Verification items for the finished model (mm, model axes). A direction names the side the tool comes from. Give positions to 0.01 mm unless a question says otherwise; leave off trailing zeros. One line per question, with ' | ' between items. Start each with the question number.
Q1. Go/stop test with flat-tipped pins: pin 1 (10 mm diameter, centred on y = 27.5, z = 22, fed in from +X); pin 2 (3 mm diameter, centred on x = -14.14, y = 14.14, fed in from +Z); pin 3 (1 mm diameter, centred on x = -38, z = 39.5, fed in from +Y). Record where each tip stops, or that it passes through.
Q2. Section check A-A on z = 7. Give the number of separate pieces and of enclosed holes in the cut face, plus the area to 3 significant figures.
Q3. Access from +Z, -Z, +X, -X, +Y, -Y to the whole of each face (thin tool, end or side, straight path). Record for faces 1 (the cylindrical face through (-47.44, 0.07, 42.35)), 2 (the cylindrical face through (14.985, 0.66, 12.325)), 3 (the flat face through (-22, -6, 2.667)), 4 (the cylindrical face through (-32, 0, 41)), 5 (the flat face through (47, 15, 27.04)).
Q4. Material ranges on probe 1 along Y at (x, z) = (0, 1); probe 2 along Y at (x, z) = (0, 5); probe 3 along X at (y, z) = (-4, 46), recorded low to high. Write a range as [from, to].
Q5. Mould release check, pull along X, two halves, no side actions. Record for faces 6 (the cylindrical face through (28, 45, 17)), 7 (the cylindrical face through (-15.362, -14.413, 21.303)), 8 (the flat face through (39, -32, 14.826)), 9 (the conical face through (14.13, 14.36, 16.88)): released by +X, released by -X, zero draft, split by the parting line, or undercut.
from build123d import *

# Parameters (mm, degrees)
SKETCH1_R                      = 53
BOSS_EXTRUDE1_DEPTH            = 50
F_10_0_10_DIAMETER_HOLE1_D     = 10
F_10_0_10_DIAMETER_HOLE1_DEPTH = 17.5
F_10_0_10_DIAMETER_HOLE1_TIP   = 3.004303095
M4_TAPPED_HOLE1_REACH          = 130.627
M4_TAPPED_HOLE1_BORE_R         = 1.65
CIRPATTERN1_COUNT              = 3
CIRPATTERN1_ANGLE              = 180
SKETCH11_R                     = 30
CUT_EXTRUDE2_DEPTH             = 25
SKETCH12_W                     = 4.826
SKETCH12_H                     = 2.76515
SKETCH12_W_2                   = 7.2136
SKETCH12_H_2                   = 4.27264
SKETCH14_W                     = 2.667
SKETCH14_H                     = 4.572
CUT_EXTRUDE3_REACH             = 92.1
SKETCH15_R                     = 15
CIRPATTERN2_COUNT              = 8
CIRPATTERN3_COUNT              = 4


with BuildPart() as part:
    # Sketch1 → Boss-Extrude1 (new body)
    with BuildSketch(Plane.XY):
        Circle(SKETCH1_R)
    extrude(amount=BOSS_EXTRUDE1_DEPTH)

    # Ø10.0 (10) Diameter Hole1
    with Locations(Plane.XY.offset(50)):
        with Locations((-37, 0), (37, 0), (0, -40)):
            Hole(F_10_0_10_DIAMETER_HOLE1_D / 2, depth=F_10_0_10_DIAMETER_HOLE1_DEPTH)
            with Locations((0, 0, -(F_10_0_10_DIAMETER_HOLE1_DEPTH + F_10_0_10_DIAMETER_HOLE1_TIP / 2))):  # 118° drill point
                Cone(0, F_10_0_10_DIAMETER_HOLE1_D / 2, F_10_0_10_DIAMETER_HOLE1_TIP, mode=Mode.SUBTRACT)

    # M4 Tapped Hole1 bore → M4 Tapped Hole1 (cut, up to next)
    with BuildSketch(Plane.ZY.offset(53), mode=Mode.PRIVATE) as m4_tapped_hole1_sk1:
        with Locations((44, 0)):
            Circle(M4_TAPPED_HOLE1_BORE_R)
    m4_tapped_hole1_tool1 = extrude(m4_tapped_hole1_sk1.sketch, amount=-M4_TAPPED_HOLE1_REACH, mode=Mode.PRIVATE) & part.part
    m4_tapped_hole1 = m4_tapped_hole1_tool1.solids().sort_by_distance((-53, 0, 44))[0]
    add(m4_tapped_hole1, mode=Mode.SUBTRACT)

    # CirPattern1: M4 Tapped Hole1 ×3 about axis
    cirpattern1_axis = Axis((0, 0, 50), (0, 0, 1))
    for i in range(1, CIRPATTERN1_COUNT):
        add(m4_tapped_hole1.rotate(cirpattern1_axis, i * CIRPATTERN1_ANGLE / (CIRPATTERN1_COUNT - 1)), mode=Mode.SUBTRACT)

    # Sketch11 → Cut-Extrude2 (cut)
    with BuildSketch(Plane.XY.offset(50)):
        Circle(SKETCH11_R)
    extrude(amount=-CUT_EXTRUDE2_DEPTH, mode=Mode.SUBTRACT)

    # Sketch12 → Cut-Revolve1 (revolve, cut)
    with BuildSketch(Plane(origin=(0, 0, 0), x_dir=(0, 0, -1), z_dir=(1, 0, 0)), mode=Mode.PRIVATE) as cut_revolve1_sk:
        with Locations((-12.413, 51.617425)):
            Rectangle(SKETCH12_W, SKETCH12_H)
        with Locations((-23.4328, 50.86368)):
            Rectangle(SKETCH12_W_2, SKETCH12_H_2)
    revolve(cut_revolve1_sk.sketch.rotate(Axis((0, 0, 0), (0, 0, 1)), 90), axis=Axis((0, 0, 0), (0, 0, 1)), mode=Mode.SUBTRACT)

    # Sketch14 → Cut-Revolve2 (revolve, cut)
    with BuildSketch(Plane(origin=(0, 0, 0), x_dir=(0, 0, -1), z_dir=(1, 0, 0)), mode=Mode.PRIVATE) as cut_revolve2_sk:
        with Locations((-1.3335, 24.8666)):
            Rectangle(SKETCH14_W, SKETCH14_H)
    revolve(cut_revolve2_sk.sketch.rotate(Axis((0, 0, 0), (0, 0, -1)), 270), axis=Axis((0, 0, 0), (0, 0, -1)), mode=Mode.SUBTRACT)

    # Sketch15 → Cut-Extrude3 (cut, up to next)
    with BuildSketch(Plane(origin=(0, 0, 0), x_dir=(-1, 0, 0), z_dir=(0, 0, -1)), mode=Mode.PRIVATE) as cut_extrude3_sk1:
        Circle(SKETCH15_R)
    cut_extrude3_tool1 = extrude(cut_extrude3_sk1.sketch, amount=-CUT_EXTRUDE3_REACH, mode=Mode.PRIVATE) & part.part
    add(cut_extrude3_tool1.solids().sort_by_distance((0, 0, 0))[0], mode=Mode.SUBTRACT)

    # Sketch17 → M5 Tapped Hole1 (revolve, cut)
    with BuildSketch(Plane(origin=(-28.284271247, 28.284271247, 0), x_dir=(0, 1, 0), z_dir=(1, 0, 0))):
        Polygon((0, 0), (0, 15.2618073), (2.1, 14), (2.1, 0), align=None)
    m5_tapped_hole1 = revolve(axis=Axis((-28.284271247, 28.284271247, -6.35), (0, 0, 1)), mode=Mode.SUBTRACT)

    # CirPattern2: M5 Tapped Hole1 ×8 about axis
    cirpattern2_axis = Axis((0, 0, 0), (0, 0, 1))
    for i in range(1, CIRPATTERN2_COUNT):
        add(m5_tapped_hole1.rotate(cirpattern2_axis, i * 360 / CIRPATTERN2_COUNT), mode=Mode.SUBTRACT)

    # Sketch19 → M3 Tapped Hole1 (revolve, cut)
    with BuildSketch(Plane(origin=(14.142135624, 14.142135624, 25), x_dir=(0, -1, 0), z_dir=(1, 0, 0))):
        Polygon((0, 0), (0, 8.251075774), (1.25, 7.5), (1.25, 0), align=None)
    m3_tapped_hole1 = revolve(axis=Axis((14.142135624, 14.142135624, 31.35), (0, 0, -1)), mode=Mode.SUBTRACT)

    # CirPattern3: M3 Tapped Hole1 ×4 about axis
    cirpattern3_axis = Axis((0, 0, 0), (0, 0, 1))
    for i in range(1, CIRPATTERN3_COUNT):
        add(m3_tapped_hole1.rotate(cirpattern3_axis, i * 360 / CIRPATTERN3_COUNT), mode=Mode.SUBTRACT)


solid = part.part
Filled in:
1) pin 1: x = 47.75 | pin 2: z = 25 | pin 3: y = 37.45
2) separate pieces: 1 | enclosed holes: 9 | area: 8,010 mm²
3) face 1: -X | face 2: +Z, -Z | face 3: -Z | face 4: +Z | face 5: none
4) probe 1: [-53, -42.1], [-37.9, -27.15], [-22.58, -15], [15, 22.58], [27.15, 37.9], [42.1, 53] | probe 2: [-53, -42.1], [-37.9, -15], [15, 37.9], [42.1, 53] | probe 3: [-52.85, -40], [-34, -29.73], [29.73, 34], [40, 52.85]
5) face 6: split by the parting line | face 7: undercut | face 8: zero draft | face 9: undercut
